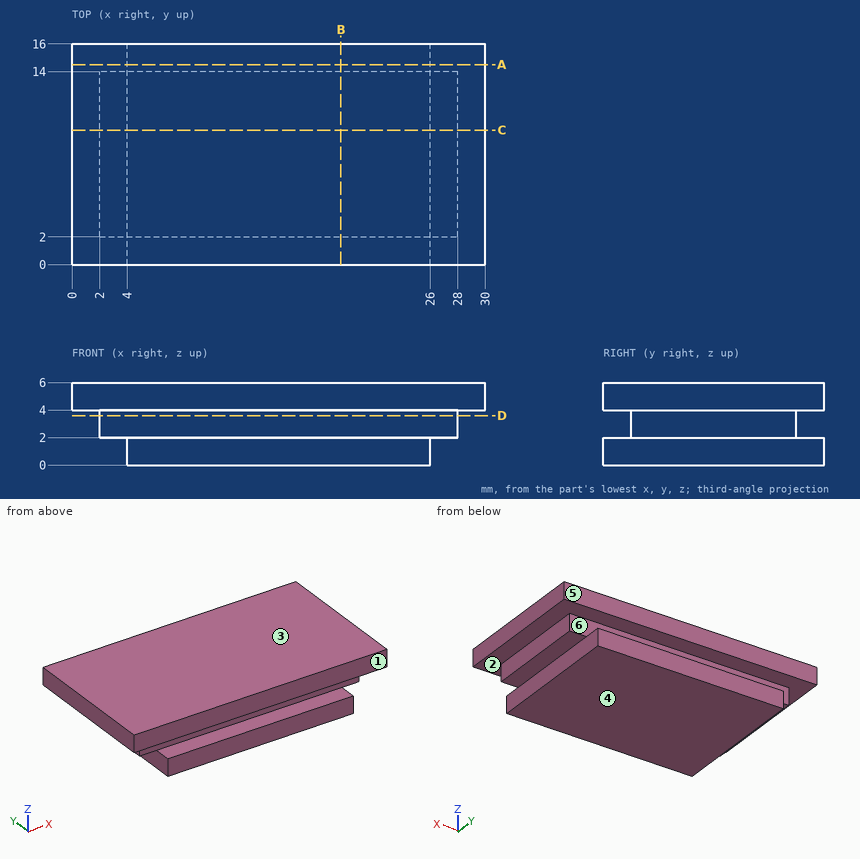
Verification items for this drawing (mm, ordinates from the low corner). A direction names the side the tool comes from. Round coordinates to 2 decimals unless told otherwise and drop trailing zeros. Order: outer loops, then holes, each group sorted by start corner. A loop starts at its lowest first (then second) coordinate and runs counter-clockwise, first axis right, second up. Notation, with made-up numbers: (69, -13.75) -> (117, -13.75) arc R35 ccw to (117, 25.25) -> close; hole circle Ø7 at (-17, -25). An arc over 180 degrees is marked (long way). Use one line per item in the form item = value.
1. Cross-section at B-B, the plane x = 19.5. Enter the section's corners in (y, z), plus the area to 3 significant figures.
Working result:
outline = (0, 0) -> (16, 0) -> (16, 2) -> (14, 2) -> (14, 4) -> (16, 4) -> (16, 6) -> (0, 6) -> (0, 4) -> (2, 4) -> (2, 2) -> (0, 2) -> close
area = 88.0 mm^2
2. Cross-section at A-A, the plane y = 14.5. Enter the section's corners in (x, z), plus the area to 3 significant figures.
Working result:
outline = (0, 4) -> (30, 4) -> (30, 6) -> (0, 6) -> close; (4, 0) -> (26, 0) -> (26, 2) -> (4, 2) -> close
area = 104 mm^2
3. Cross-section at C-C, the plane y = 9.75. Enter the section's corners in (x, z), plus the area to 3 significant figures.
Working result:
outline = (0, 4) -> (2, 4) -> (2, 2) -> (4, 2) -> (4, 0) -> (26, 0) -> (26, 2) -> (28, 2) -> (28, 4) -> (30, 4) -> (30, 6) -> (0, 6) -> close
area = 156 mm^2
4. Mould release check, pull along Z, two halves, no side actions. Record for the marked faces 1, 2, 3 and 4: pulls with the +Z half, pulls with the -Z half, needs draft (parallel to the pull), parting line crosses it, or undercut.
Working result:
face_1 = needs draft
face_2 = undercut
face_3 = pulls with the +Z half
face_4 = pulls with the -Z half
5. Set-up check for the marked faces 5 and 6: record each of +Z, -Z, +X, -X, +Y, -Y from which the full face is reachable in a straight line by a thin tool's end or side.
Working result:
face_5 = +Z, -Z, +X, -X, +Y
face_6 = +X, -X, +Y
6. Scan lines: line 1 along Z through (x, y) = (6.75, 1.75); line 2 along X through (y, z) = (3.5, 3.7); line 3 along X through (y, z) = (1.25, 0.5). Record each from-to range of solid material in increasing order. Write a range as from..to.
Working result:
line_1 = 0..2, 4..6
line_2 = 2..28
line_3 = 4..26
7. Go/stop test with flat-tipped pins: pin 1 (1 mm diameter, centred on x = 3, y = 11, fed in from -Z); pin 2 (1 mm diameter, centred on x = 10, z = 3, fed in from +Y); pin 3 (1 mm diameter, centred on y = 8, z = 0.5, fed in from +X). Record where each tip stops, or that it passes through.
Working result:
pin_1 = 2
pin_2 = 14
pin_3 = 26
8. Cross-section at D-D, the plane z = 3.6. Enter the section's corners in (x, y), plus the area to 3 significant figures.
Working result:
outline = (2, 2) -> (28, 2) -> (28, 14) -> (2, 14) -> close
area = 312 mm^2
